Work out the finished part from the listing and answer in its coordinate system (mm). A direction names the side the tool comes from. Give positions to 0.01 mm unless a question says otherwise; leave off trailing zeros. Loops run counter-clockwise (first coordinate to the right, second up) from the corner with the lowest first, then second, coordinate; pieces in that order, holes last. Notation, with made-up numbers: (-6, 41.5) - (-2, 41.5) arc R13 cw to (-2, 45.5) - close; hole circle Ø4 at (76.5, 1.25). An arc over 180 degrees is marked (long way). Use one line per item in the form item = value. Start each with the question number.
Autodesk Inventor part; units mm, degrees
ref_plane "MidSidePlane" through (0, 10, 0) normal (0, 1, 0) x (-1, 0, 0)
ref_plane "YZ Plane" through (0, 0, 0) normal (1, 0, 0) x (0, 1, 0)
ref_plane "XY Plane" through (0, 0, 0) normal (0, 0, 1) x (1, 0, 0)
sketch "Mount" plane through (0, 0, 0) normal (0, 0, 1) x (1, 0, 0)
  circle A0 centre (0, 0) radius 9.5
  dimension "d0" = 19
extrude "MountFeature" add sketch "Mount" along normal blind 8
sketch "Base" plane through (0, 0, 8) normal (0, 0, 1) x (1, 0, 0)
  circle A0 centre (0, 0) radius 9.5 construction
  circle A1 centre (0, 0) radius 11
  dimension "d3" = 22
extrude "BaseFeature" add sketch "Base" along normal blind 3
chamfer "BaseChamferFeature" distance 1 angle 45 1 edges at (-11, 0, 11)
sketch "RodEndHole" plane through (0, 0, 11) normal (0, 0, 1) x (1, 0, 0)
  circle A0 centre (0, 0) radius 10 construction
hole "RodEndHoleFeature" at (0, 0, 11) direction (0, 0, -1) diameter 4.978 end through all
ref_plane "MidSidePlane" through (0, 10, 0) normal (0, 1, 0) x (-1, 0, 0)
sketch "MountHole" plane through (0, 10, 0) normal (0, 1, 0) x (-1, 0, 0)
  line L0 (-11, 8) -> (11, 8) construction
  line L1 (-9.5, 0) -> (-9.5, 8) construction
  point P0 (0, 3.5)
  dimension "d18" = 4.5
  dimension "d26" = 22
  dimension "d27" = 11
hole "MountHoleFeature" at (0, 10, 3.5) direction (0, -1, 0) diameter 2.459 end through all
properties part number "BackPair1PistonTopCap"
1) A cutting plane is placed at B-B (z = 3.5). Give the vertices of the cut face in (x, y).
2) A cutting plane is placed at C-C (x = 0). Give the vertices of the cut face in (y, z).
3) Flat-ended cylindrical pins translate along their axes: pin 1 Ø4.5 at (x, y) = (0, 0) entering from +Z; pin 2 Ø1 at (y, z) = (-2.5, 8) entering from -X; pin 3 Ø5 at (y, z) = (-6.5, 3.5) entering from -X. Find the tip coordinate at first contact, or state that the pin passes through.
4) Determine the mould class of faces 3 (the cylindrical face through (-0.05, 5.78, 2.27)), 4 (the cylindrical face through (-2.38, 10.74, 8.99)), 5 (the flat face through (-10, 0, 8)) for opening direction X: released by +X, released by -X, zero draft, split by the parting line, or undercut.
5) A tool of negligible diameter and unlimited length cuts with its end or side. For faces 1 (the cylindrical face through (4.38, 8.43, 3.94)), 2 (the cylindrical face through (-0.05, -5.88, 2.27)), from which of +Z, -Z, +X, -X, +Y, -Y can it reach the whole face along a straight path? Write none if from no direction.
6) Find the intervals of material crossed by probe 1 along Z at (x, y) = (0, 6.5); probe 2 along Y at (x, z) = (0, 6); probe 3 along Y at (x, z) = (-1.25, 6.5), in increasing order.
7) A cutting plane is placed at D-D (z = 1.25). Give the vertices of the cut face in (x, y).
8) A cutting plane is placed at A-A (y = 0). Give the vertices of the cut face in (x, z).
Answer sheet:
q1.outline = (-1.23, -9.42) - (-1.23, -2.16) arc R2.49 cw to (-1.23, 2.16) - (-1.23, 9.42) arc R9.5 ccw to start; (1.23, -9.42) arc R9.5 ccw to (1.23, 9.42) - (1.23, 2.16) arc R2.49 cw to (1.23, -2.16) - close
q2.outline = (-11, 8) - (-9.5, 8) - (-9.5, 4.73) - (-2.49, 4.73) - (-2.49, 11) - (-10, 11) - (-11, 10) - close; (-9.5, 0) - (-2.49, 0) - (-2.49, 2.27) - (-9.5, 2.27) - close; (2.49, 0) - (9.5, 0) - (9.5, 2.27) - (2.49, 2.27) - close; (2.49, 4.73) - (9.5, 4.73) - (9.5, 8) - (11, 8) - (11, 10) - (10, 11) - (2.49, 11) - close
q3.pin_1 = through
q3.pin_2 = -10.82
q3.pin_3 = -8.62
q4.face_3 = undercut
q4.face_4 = split by the parting line
q4.face_5 = zero draft
q5.face_1 = -Z
q5.face_2 = +Y, -Y
q6.probe_1 = 0 to 2.27, 4.73 to 11
q6.probe_2 = -9.5 to -2.49, 2.49 to 9.5
q6.probe_3 = -9.42 to -2.15, 2.15 to 9.42
q7.outline = circle Ø19 at (0, 0); hole circle Ø4.98 at (0, 0)
q8.outline = (-11, 8) - (-9.5, 8) - (-9.5, 0) - (-2.49, 0) - (-2.49, 11) - (-10, 11) - (-11, 10) - close; (2.49, 0) - (9.5, 0) - (9.5, 8) - (11, 8) - (11, 10) - (10, 11) - (2.49, 11) - close
